Autodesk Inventor part; units mm, degrees
ref_plane "YZ Plane" through (0, 0, 0) normal (1, 0, 0) x (0, 1, 0)
ref_plane "XZ Plane" through (0, 0, 0) normal (0, 1, 0) x (-1, 0, 0)
ref_plane "XY Plane" through (0, 0, 0) normal (0, 0, 1) x (1, 0, 0)
sketch "スケッチ4" plane through (0, 0, 0) normal (1, 0, 0) x (0, 1, 0)
  line L0 (0, 0) -> (0, -100)
  line L1 (0, -50) -> (-20, -50)
  arc A0 (0, 0) -> (0, -100) centre (52.5, -50) ccw
  dimension "d23" = 100
  dimension "d24" = 20
extrude "押し出し3" add sketch "スケッチ4" against normal blind 10
sketch "スケッチ5" plane through (0, 0, 0) normal (1, 0, 0) x (0, 0, -1)
  line L0 (40, 130) -> (60, 130)
  line L1 (60, 130) -> (60, 0)
  line L2 (60, 0) -> (40, 0)
  line L3 (40, 0) -> (40, 130)
  line L4 (100, 0) -> (0, 0)
  point P0 (50, 0)
  point P1 (50, 0)
  dimension "d27" = 20
  dimension "d28" = 130
  dimension "d29" = 0
  dimension "d30" = 0
extrude "押し出し4" add sketch "スケッチ5" against normal blind 4
sketch "スケッチ6" plane through (0, 0, 0) normal (1, 0, 0) x (0, 0, -1)
  line L0 (60, 0) -> (60, 130)
  line L1 (60, 130) -> (40, 130)
  point P0 (0, 0)
  point P1 (50, 120)
  dimension "d33" = 10
  dimension "d34" = 10
hole "穴2" at (0, 120, -50) direction (-1, 0, 0) diameter 10 end through all
sketch "スケッチ7" plane through (0, 0, 0) normal (1, 0, 0) x (0, 0, -1)
  line L0 (40, 0) -> (60, 0)
  line L1 (60, 0) -> (60, 130)
  point P0 (0, 0)
  point P1 (52.5, -9.6825)
  point P2 (50, 0)
  dimension "d42" = 10
  dimension "d43" = 7.5
hole "穴3" at (0, -9.6825, -52.5) direction (-1, 0, 0) diameter 6 end through all counterbore diameter 10 counterbore depth 5
fillet "フィレット1" radius 7.5 2 edges at (-2, 130, -40) (-2, 130, -60)
fillet "フィレット2" radius 2 3 edges at (-2, 0, -40) (-4, 0, -50) (-2, 0, -60)
fillet "フィレット3" radius 2 2 edges at (-5, 0, 0) (-5, 0, -100)
properties part number "受動歩行_ver3"
The listing builds one solid part. Answer for the finished solid, in the listing's coordinates (mm). A direction names the side the tool comes from. Give positions to 0.01 mm unless a question says otherwise; leave off trailing zeros. Order: outer loops, then holes, each group sorted by start corner. A loop starts at its lowest first (then second) coordinate and runs counter-clockwise, first axis right, second up. Notation, with made-up numbers: (63, 24) -> (84, 24) arc R24 cw to (84, 39) -> close; hole circle Ø10 at (58, 76). An arc over 180 degrees is marked (long way). Answer as CSV lines item,"result". Start each with the question number.
Q1. Find the intervals of material crossed by L1, parallel to Y at x = -2.8, z = -52.5; L2, parallel to Z at x = -3.5, y = 43.5; L3, parallel to Z at x = -3.25, y = -9, in increasing order.
Q2. Given pin 1 (3 mm diameter, centred on y = -12, z = -54, fed in from +X); pin 2 (1.2 mm diameter, centred on x = -1, y = 70.5, fed in from -Z); pin 3 (1.5 mm diameter, centred on x = -4, z = -44.5, fed in from +Y), each flat-ended and moving along its own axis, determine where each tip first touches the part or whether it passes through.
Q3. A cutting plane is placed at C-C (x = -2). Determine the outline of the cut face in (y, z).
Q4. Which of the six approach directions +Z, -Z, +X, -X, +Y, -Y give full straight-line access (tool end or side, diameter ignored) to faces 5 (the flat face through (-5, -10, -56)), 6 (the flat face through (-7, 0, -49)), 7 (the flat face through (-4, 67, -50)), 8 (the flat face through (-2, 63, -60))?
Q5. Determine the mould class of faces 1 (the flat face through (-2, 61, -40)), 2 (the cylindrical face through (-2.028, 127.861, -57.745)), 3 (the cylindrical face through (-2, 117, -46)), 4 (the cylindrical face through (-4.93, -19.997, -49.303)) for opening direction Y: pulls with the +Y half, pulls with the -Y half, needs draft (parallel to the pull), parting line crosses it, or undercut.
Q6. A cutting plane is placed at B-B (z = -43). Determine the outline of the cut face in (x, y).
Q7. A cutting plane is placed at D-D (y = 6). Determine the outline of the cut face in (x, z).
Q8. A cutting plane is placed at A-A (y = 120). Determine the outline of the cut face in (x, z).
Results found:
1,L1,"-19.96 to -14.68, -4.68 to 115.67, 124.33 to 130"
1,L2,"-60 to -40"
1,L3,"-88.39 to -57.45, -47.55 to -11.61"
2,pin 1,"x = -5"
2,pin 2,"z = -60"
2,pin 3,"y = 129.65"
3,outline,"(-3.55, -95.99) arc R2 ccw to (0, -94.72) -> (0, -62) arc R2 cw to (2, -60) -> (122.5, -60) arc R7.5 ccw to (130, -52.5) -> (130, -47.5) arc R7.5 ccw to (122.5, -40) -> (2, -40) arc R2 cw to (0, -38) -> (0, -5.28) arc R2 ccw to (-3.55, -4.01) arc R72.5 ccw to start; hole circle Ø10 at (-9.68, -52.5); hole circle Ø10 at (120, -50)"
4,face 5,"+X"
4,face 6,"-X, +Y"
4,face 7,"+Z, -Z, -X, +Y"
4,face 8,"-Z, +X, -X, +Y"
5,face 1,"needs draft"
5,face 2,"pulls with the +Y half"
5,face 3,"undercut"
5,face 4,"pulls with the -Y half"
6,outline,"(-10, -19.66) -> (0, -19.66) -> (0, 128.5) -> (-4, 128.5) -> (-4, 2) arc R2 cw to (-6, 0) -> (-10, 0) -> close"
7,outline,"(-4, -60) -> (0, -60) -> (0, -40) -> (-4, -40) -> close"
8,outline,"(-4, -60) -> (0, -60) -> (0, -55) -> (-4, -55) -> close; (-4, -45) -> (0, -45) -> (0, -40) -> (-4, -40) -> close"
